Source: CAD feature listing. Evaluate the final solid. Frame: model axes, mm. A direction names the side the tool comes from. Round coordinates to 2 decimals unless told otherwise and drop trailing zeros. Loops run counter-clockwise (first coordinate to the right, second up) from the corner with the lowest first, then second, coordinate; pieces in that order, holes last. Notation, with made-up numbers: M -30,11.25 L 5,11.25 A34 ccw 5,43.25 Z; hole C 67,55.5 d11. An arc over 180 degrees is marked long. One line per item, written item: value.
from build123d import *

# Parameters (mm, degrees)
F0_R      = 298.45
F1_DEPTH  = 152.4
F11_W     = 1267.8290780676
F11_H     = 1016
F16_DEPTH = 76.2


with BuildPart() as f1:
    # F0 (on Top) → F1 (new body)
    with BuildSketch(Plane.XY):
        with BuildLine():
            ThreePointArc((272.9734828671, 135.6042685589), (263.9645430735, 152.4), (253.9234828671, 168.599836443))
            ThreePointArc((253.9234828671, 168.599836443), (152.4, 263.9645430735), (19.05, 304.2041050019))
            ThreePointArc((19.05, 304.2041050019), (9.5296588455, 304.6509898265), (0, 304.8))
            ThreePointArc((0, 304.8), (-9.5296588455, 304.6509898265), (-19.05, 304.2041050019))
            ThreePointArc((-19.05, 304.2041050019), (-152.4, 263.9645430735), (-253.9234828671, 168.599836443))
            ThreePointArc((-253.9234828671, 168.599836443), (-263.9645430735, 152.4), (-272.9734828671, 135.6042685589))
            ThreePointArc((-272.9734828671, 135.6042685589), (-304.8, 0), (-272.9734828671, -135.6042685589))
            ThreePointArc((-272.9734828671, -135.6042685589), (-268.6003259006, -144.0725682636), (-263.9645430735, -152.4))
            ThreePointArc((-263.9645430735, -152.4), (-259.0706670551, -160.5784215629), (-253.9234828671, -168.599836443))
            ThreePointArc((-253.9234828671, -168.599836443), (-152.4, -263.9645430735), (-19.05, -304.2041050019))
            ThreePointArc((-19.05, -304.2041050019), (0, -304.8), (19.05, -304.2041050019))
            ThreePointArc((19.05, -304.2041050019), (152.4, -263.9645430735), (253.9234828671, -168.599836443))
            ThreePointArc((253.9234828671, -168.599836443), (259.0706670551, -160.5784215629), (263.9645430735, -152.4))
            ThreePointArc((263.9645430735, -152.4), (268.6003259006, -144.0725682636), (272.9734828671, -135.6042685589))
            ThreePointArc((272.9734828671, -135.6042685589), (296.7367162805, -69.6445346818), (304.8, 0))
            ThreePointArc((304.8, 0), (296.7367162805, 69.6445346818), (272.9734828671, 135.6042685589))
        make_face()
        Circle(F0_R, mode=Mode.SUBTRACT)
    extrude(amount=-F1_DEPTH)

    # F2 (on Front) → F9 (revolve)
    with BuildSketch(Plane.XZ):
        with BuildLine():
            Line((0, -447.3894571287), (0, -453.7394571287))
            ThreePointArc((0, -453.7394571287), (214.306152748, -365.6868034652), (304.8, -152.4))
            Line((304.8, -152.4), (294.9894571287, -152.4))
            ThreePointArc((294.9894571287, -152.4), (208.5890455143, -360.9890455142), (0, -447.3894571287))
        make_face()
    revolve(axis=Axis((0, 0, -248.1805924326), (0, 0, -1)))

    # F8 (on face) → F12 (revolve)
    with BuildSketch(Plane(origin=(0, 0, 0), x_dir=(0, -1, 0), z_dir=(-1, 0, 0))):
        with BuildLine():
            Line((-201.9116809095, -377.2763831548), (-304.8, -609.6))
            Line((-304.8, -609.6), (-271.7425017268, -609.6))
            Line((-271.7425017268, -609.6), (-177.4761269208, -396.7448835454))
            ThreePointArc((-177.4761269208, -396.7448835454), (-189.9434989923, -387.3239083256), (-201.9116809095, -377.2763831548))
        make_face()
    revolve(axis=Axis((0, 136.6116201303, -304.4721153432), (0, 0.4049332191, -0.9143462627)))

    # F7 (on face) → F13 (revolve)
    with BuildSketch(Plane(origin=(0, 0, 0), x_dir=(-0.8660254038, 0.5, 0), z_dir=(0.5, 0.8660254038, 0))):
        with BuildLine():
            Line((-201.9116809095, -377.2763831548), (-304.8, -609.6))
            Line((-304.8, -609.6), (-271.7425017268, -609.6))
            Line((-271.7425017268, -609.6), (-177.4761269208, -396.7448835454))
            ThreePointArc((-177.4761269208, -396.7448835454), (-189.9434989923, -387.3239083256), (-201.9116809095, -377.2763831548))
        make_face()
    revolve(axis=Axis((118.309133485, -68.3058100652, -304.4721153432), (0.3506824545, -0.2024666095, -0.9143462627)))

    # F6 (on face) → F14 (revolve)
    with BuildSketch(Plane(origin=(0, 0, 0), x_dir=(0.8660254038, 0.5, 0), z_dir=(0.5, -0.8660254038, 0))):
        with BuildLine():
            Line((-201.9116809095, -377.2763831548), (-304.8, -609.6))
            Line((-304.8, -609.6), (-271.7425017268, -609.6))
            Line((-271.7425017268, -609.6), (-177.4761269208, -396.7448835454))
            ThreePointArc((-177.4761269208, -396.7448835454), (-189.9434989923, -387.3239083256), (-201.9116809095, -377.2763831548))
        make_face()
    revolve(axis=Axis((-118.309133485, -68.3058100652, -304.4721153432), (-0.3506824545, -0.2024666095, -0.9143462627)))

    # F2 (on Front) → F15 (revolve, cut)
    with BuildSketch(Plane.XZ):
        with BuildLine():
            Line((0, -152.4), (0, -447.3894571287))
            ThreePointArc((0, -447.3894571287), (208.5890455143, -360.9890455142), (294.9894571287, -152.4))
            Line((294.9894571287, -152.4), (0, -152.4))
        make_face()
    revolve(axis=Axis((0, 0, -248.1805924326), (0, 0, -1)), mode=Mode.SUBTRACT)

    # F11 (on offset) → F16 (cut)
    with BuildSketch(Plane.XY.offset(-609.6)):
        with Locations((7.6045542955, -77.3831754923)):
            Rectangle(F11_W, F11_H)
    extrude(amount=-F16_DEPTH, mode=Mode.SUBTRACT)


solid = f1.part
1. Ray query, line 1 (Y direction, x = 0, z = -87); line 2 (Y direction, x = -109.5, z = -31.5); line 3 (X direction, y = 170, z = -123). Return the intervals inside material, ascending. Write a range as [from, to].
Report:
line 1: y = [-304.8, -298.45], [298.45, 304.8]
line 2: y = [-284.45, -277.64], [277.64, 284.45]
line 3: x = [-252.99, -245.3], [245.3, 252.99]
2. Pin query (flat end, axial travel): pin 1 (6 mm diameter, centred on x = -98, y = 217, fed in from +Z); pin 2 (1 mm diameter, centred on y = 154, z = -205, fed in from -X); pin 3 (5 mm diameter, centred on y = -221.5, z = -297.5, fed in from -X). Return the tip coordinate at first contact, or that it passes through.
Report:
pin 1: stops at z = -322.37
pin 2: stops at x = -257.33
pin 3: stops at x = -152
3. Pull-direction query (Z, two-part tool) for faces 3 (the face through (-223.47, -118.54, -495.63)), 4 (the face through (224, -202, 0)), 5 (the face through (235, -135, -609.6)); classes: released by +Z, released by -Z, zero draft, split by the parting line, or undercut.
Report:
face 3: undercut
face 4: released by +Z
face 5: released by -Z
4. Section query A-A (y = -44). Return the cut outline in (x, z), and give its area (3 significant figures).
Report:
outline: M -301.61,-152.4 A301.63 ccw 301.61,-152.4 L 301.61,0 L 295.19,0 L 295.19,-152.4 L 291.69,-152.4 A291.69 cw -291.69,-152.4 L -295.19,-152.4 L -295.19,0 L -301.61,0 Z
area: 9,120 mm2
5. Section query B-B (x = -49.5). Return the cut outline in (y, z), and give its area (3 significant figures).
Report:
outline: M -300.75,-152.4 A300.77 ccw 300.75,-152.4 L 300.75,0 L 294.32,0 L 294.32,-152.4 L 290.81,-152.4 A290.81 cw -290.81,-152.4 L -294.32,-152.4 L -294.32,0 L -300.75,0 Z
area: 9,130 mm2
6. Reachability of faces 1 (the face through (-289, -68, -152.4)), 2 (the face through (0, 272, -609.6)) from +Z, -Z, +X, -X, +Y, -Y: full face, straight path, thin tool, end or side. Return the list, or none.
Report:
face 1: +Z
face 2: -Z, +X, -X, +Y, -Y
7. Section query C-C (z = -218). Return the cut outline in (x, y).
Report:
outline: C 0,0 d593.78; hole C 0,0 d575.21
8. Section query D-D (z = -539). Count the separate pieces of the cut face and the enclosed holes in it, and give its area (3 significant figures).
Report:
separate pieces: 3
enclosed holes: 0
area: 9,420 mm2
